Here's how the part is built. I have some questions about the finished solid (model axes, mm). A direction names the side the tool comes from. Give positions to 0.01 mm unless a question says otherwise; leave off trailing zeros. Write each loop counter-clockwise with the first axis right and the second up, starting at its lowest first coordinate (ties: lowest second). Pieces come first, ordered by that corner, then holes. Notation, with made-up numbers: (11, 14.5) -> (58, 14.5) arc R12 cw to (58, 35.5) -> close; hole circle Ø9 at (89.25, 34.25). An arc over 180 degrees is marked (long way). Use one line per item in the form item = value.
```python
from build123d import *

# Parameters (mm, degrees)
SKETCH1_W           = 37
SKETCH1_H           = 55
BOSS_EXTRUDE1_DEPTH = 6
SKETCH2_W           = 4.36600783
SKETCH2_H           = 10.66713821
SKETCH2_H_2         = 12.422520393
SKETCH2_H_3         = 11.48339845
CUT_EXTRUDE1_DEPTH  = 67.558245169
FILLET1_R           = 7


with BuildPart() as part:
    # Sketch1 → Boss-Extrude1 (new body)
    with BuildSketch(Plane(origin=(0, 0, 0), x_dir=(1, 0, 0), z_dir=(0, 1, 0))):
        with Locations((18.5, 27.5)):
            Rectangle(SKETCH1_W, SKETCH1_H)
    extrude(amount=BOSS_EXTRUDE1_DEPTH)

    # Sketch2 → Cut-Extrude1 (cut, through all)
    with BuildSketch(Plane(origin=(0, 6, 0), x_dir=(1, 0, 0), z_dir=(0, 1, 0))):
        with Locations((34.816996085, 49.666430895)):
            Rectangle(SKETCH2_W, SKETCH2_H)
        with Locations((34.816996085, 30.703899365)):
            Rectangle(SKETCH2_W, SKETCH2_H_2)
        with Locations((34.816996085, 5.741699225)):
            Rectangle(SKETCH2_W, SKETCH2_H_3)
    extrude(amount=-CUT_EXTRUDE1_DEPTH, mode=Mode.SUBTRACT)

    # Fillet1
    fillet1_edges = [part.edges().sort_by_distance(p)[0] for p in [
        (32.63399217, 3, -55),
        (32.63399217, 3, 0),
    ]]
    fillet(fillet1_edges, radius=FILLET1_R)


solid = part.part
```
Q1. If we mould it in two halves opening along Z, with no side actions, what happens to faces 1 (the face through (18, 0, -28)), 2 (the face through (35, 3, -44.333)), 3 (the face through (32.634, 3, -31)), 4 (the face through (35, 3, -36.915))? For each: +Z half, -Z half, draft (parallel to the pull), parting line (faces both ways), or undercut.
Result set:
face_1 = draft
face_2 = -Z half
face_3 = undercut
face_4 = undercut
Q2. I want a section at C-C, the plane x = 30.5. Write out the boundary of the cut face in (y, z), and give its area (3 significant figures).
Result set:
outline = (0, -53.03) -> (6, -53.03) -> (6, -1.97) -> (0, -1.97) -> close
area = 306 mm2
Q3. I want a section at B-B, the plane z = -34. Write out the boundary of the cut face in (x, y).
Result set:
outline = (0, 0) -> (32.63, 0) -> (32.63, 6) -> (0, 6) -> close
Q4. If I drill on line 1 along X through (y, z) = (1.45, -31.5); line 2 along Z through (x, y) = (30.5, 3.55); line 3 along Z through (x, y) = (28.5, 3.85), over which ranges is the centre line in solid material (lowest first)? Write a range as from..to.
Result set:
line_1 = 0..32.63
line_2 = -53.03..-1.97
line_3 = -54.39..-0.61
Q5. I want a section at A-A, the plane y = 4.7. Write out the boundary of the cut face in (x, z), and give its area (3 significant figures).
Result set:
outline = (0, -55) -> (25.63, -55) arc R7 ccw to (32.63, -48) -> (32.63, -44.33) -> (37, -44.33) -> (37, -36.92) -> (32.63, -36.92) -> (32.63, -24.49) -> (37, -24.49) -> (37, -11.48) -> (32.63, -11.48) -> (32.63, -7) arc R7 ccw to (25.63, 0) -> (0, 0) -> close
area = 1,860 mm2
Q6. Will these pins go through, and if not, where does the flat tip stop? pin 1 Ø3.5 at (x, y) = (35.5, 3) entering from +Z; pin 2 Ø3.5 at (x, y) = (35.5, 1.5) entering from -Z; pin 3 Ø1 at (x, y) = (30, 2) entering from -Z.
Result set:
pin_1 = -11.48
pin_2 = -44.33
pin_3 = -53.84
Q7. Which directions (+Z, -Z, +X, -X, +Y, -Y) give clear straight access to the entire face, cutting with the end or side of a thin tool? Please do faces 5 (the face through (35, 3, -24.493)), 6 (the face through (13, 3, 0)), 7 (the face through (32.634, 3, -46)), 8 (the face through (37, 3, -18)), 9 (the face through (32.634, 3, -9)).
Result set:
face_5 = +X, +Y, -Y
face_6 = +Z, +X, -X, +Y, -Y
face_7 = -Z, +X, +Y, -Y
face_8 = +Z, -Z, +X, +Y, -Y
face_9 = +Z, +X, +Y, -Y
